Check sheet for the drawn part. Datum: minimum x, y, z corner. Units: mm. A direction names the side the tool comes from. Coordinates: 2 decimals unless noted, no trailing zeros. Loops run counter-clockwise (first coordinate to the right, second up) from the corner with the lowest first, then second, coordinate; pieces in that order, holes last. Notation, with made-up numbers: (30.5, -20) - (55.5, -20) arc R22 cw to (55.5, -11) - close; hole circle Ø4 at (4.25, 41). An arc over 180 degrees is marked (long way). Answer as CSV lines item,"result". Start each with the question number.
1. Set-up check for the marked faces 1, 2 and 3: record each of +Z, -Z, +X, -X, +Y, -Y from which the full face is reachable in a straight line by a thin tool's end or side.
2. Cross-section at A-A (y = 55). Enter the section's corners in (x, z), plus the area to 3 significant figures.
3. Cross-section at C-C (x = 58). Enter the section's corners in (y, z).
4. Gauge pin test, flat ends, axial feed: P1, Ø1, axis at x = 102, y = 56, coming from the -Z side; P2, Ø6, axis at x = 85.5, z = 56, coming from the +Y side; P3, Ø10, axis at x = 22, y = 38, coming from the +Z side. Record the tip position at first contact, or that the pin passes through.
5. Release check for a two-part mould opening along Y. For the marked faces 4, 5 and 6 record: pulls with the +Y half, pulls with the -Y half, needs draft (parallel to the pull), parting line crosses it, or undercut.
6. Material ranges on line 1 (X direction, y = 34, z = 110.5); line 2 (Y direction, x = 31, z = 95.5); line 3 (Z direction, x = 34.5, y = 15.5), recorded low to high. Write a range as [from, to].
7. Cross-section at B-B (z = 90.5). Enter the section's corners in (x, y).
8. Cross-section at D-D (z = 77). Enter the section's corners in (x, y).
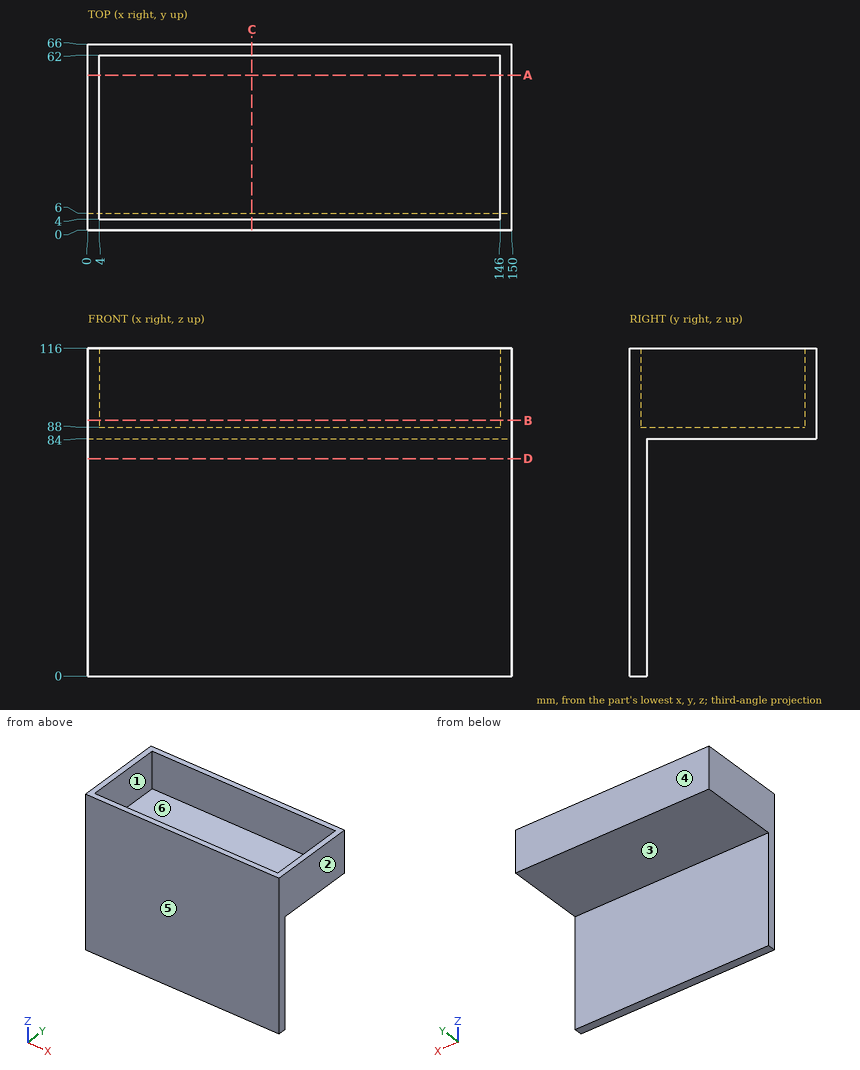
Values follow:
1,face 1,"+Z"
1,face 2,"+Z, -Z, +X, +Y, -Y"
1,face 3,"-Z, +X, -X, +Y"
2,outline,"(0, 84) - (150, 84) - (150, 116) - (146, 116) - (146, 88) - (4, 88) - (4, 116) - (0, 116) - close"
2,area,"824 mm²"
3,outline,"(0, 0) - (6, 0) - (6, 84) - (66, 84) - (66, 116) - (62, 116) - (62, 88) - (4, 88) - (4, 116) - (0, 116) - close"
4,P1,"stops at z = 84"
4,P2,"stops at y = 6"
4,P3,"stops at z = 88"
5,face 4,"pulls with the +Y half"
5,face 5,"pulls with the -Y half"
5,face 6,"undercut"
6,line 1,"x = [0, 4], [146, 150]"
6,line 2,"y = [0, 4], [62, 66]"
6,line 3,"z = [84, 88]"
7,outline,"(0, 0) - (150, 0) - (150, 66) - (0, 66) - close; hole (4, 4) - (146, 4) - (146, 62) - (4, 62) - close"
8,outline,"(0, 0) - (150, 0) - (150, 6) - (0, 6) - close"
